Read the model definition and answer for the solid it produces. Units are mm, in the model's axes. Give positions to 0.01 mm unless a question says otherwise; leave off trailing zeros. Order: outer loops, then holes, each group sorted by start corner. A loop starts at its lowest first (then second) coordinate and runs counter-clockwise, first axis right, second up. Notation, with made-up numbers: M 76.25,-4 L 105.25,-4 A29 cw 105.25,35 Z; hole C 83,13.5 d5. An arc over 180 degrees is marked long. Write item = value, one per line. Start each with the question number.
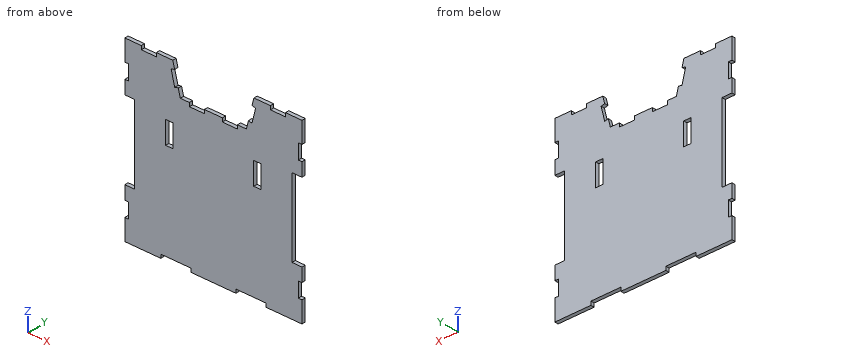
from build123d import *

# Parameters (mm, degrees)
CROQUIS1_W              = 4.84
CROQUIS1_H              = 15
SALIENTE_EXTRUIR1_DEPTH = 2.44


with BuildPart() as part:
    # Croquis1 → Saliente-Extruir1 (new body)
    with BuildSketch(Plane(origin=(0, 0, 0), x_dir=(1, 0, 0), z_dir=(0, 1, 0))):
        Polygon((-59, 45), (-59, 59), (-35, 59), (-35, 56.56), (-15, 56.56), (-15, 59), (15, 59), (15, 56.56), (35, 56.56), (35, 59), (59, 59), (59, 45), (56.56, 45), (56.56, 35), (59, 35), (59, 26), (52.4, 26), (52.4, -26), (59, -26), (59, -35), (56.56, -35), (56.56, -45), (59, -45), (59, -59), (48, -59), (48, -56.56), (38, -56.56), (38, -59), (27, -59), (25.787321875, -54.149287499), (28.154469575, -53.557500574), (25.729113325, -43.856075573), (23.361965624, -44.447862498), (22, -39), (16, -39), (16, -36.56), (6, -36.56), (6, -39), (-6, -39), (-6, -36.56), (-16, -36.56), (-16, -39), (-22, -39), (-23.361965624, -44.447862498), (-25.729113325, -43.856075573), (-28.154469575, -53.557500574), (-25.787321875, -54.149287499), (-27, -59), (-38, -59), (-38, -56.56), (-48, -56.56), (-48, -59), (-59, -59), (-59, -45), (-56.56, -45), (-56.56, -35), (-59, -35), (-59, -26), (-52.4, -26), (-52.4, 26), (-59, 26), (-59, 35), (-56.56, 35), (-56.56, 45), align=None)
        with Locations((29.32, -15.28)):
            Rectangle(CROQUIS1_W, CROQUIS1_H, mode=Mode.SUBTRACT)
        with Locations((-29.32, -15.28)):
            Rectangle(CROQUIS1_W, CROQUIS1_H, mode=Mode.SUBTRACT)
    extrude(amount=SALIENTE_EXTRUIR1_DEPTH)


solid = part.part
1) Find section C-C on x = -44.5. Determine the outline of the cut face in (y, z).
2) Find the intervals of material crossed by probe 1 along X at (y, z) = (2.15, 10); probe 2 along X at (y, z) = (0.1, 5); probe 3 along Z at (x, y) = (15.5, 1.75), in increasing order. Write a range as [from, to].
3) Find section D-D on y = 1.6. Count the separate pieces of the cut face and the enclosed holes in it, plus the area to 3 significant figures.
4) Find section A-A on x = -30. Determine the outline of the cut face in (y, z), plus the area to 3 significant figures.
5) Each of these flat-tipped pins is pushed along its axis until it touches: P1, Ø0.7, axis at x = -44.5, y = 1.5, coming from the +Z side; P2, Ø2, axis at x = 32, z = -42, coming from the -Y side; P3, Ø0.7, axis at y = 1.5, z = -41.5, coming from the -X side. Where does it stop, or does it pass through?
6) Find section B-B on z = -41. Determine the outline of the cut face in (x, y).
Numbers:
q1.outline = M 0,-59 L 2.44,-59 L 2.44,56.56 L 0,56.56 Z
q2.probe_1 = [-52.4, -31.74], [-26.9, 26.9], [31.74, 52.4]
q2.probe_2 = [-52.4, 52.4]
q2.probe_3 = [-56.56, 36.56]
q3.separate_pieces = 1
q3.enclosed_holes = 2
q3.area = 11,800 mm2
q4.outline = M 0,-56.56 L 2.44,-56.56 L 2.44,7.78 L 0,7.78 Z; M 0,22.78 L 2.44,22.78 L 2.44,59 L 0,59 Z
q4.area = 245 mm2
q5.P1 = 56.56
q5.P2 = 0
q5.P3 = -56.56
q6.outline = M -56.56,0 L 56.56,0 L 56.56,2.44 L -56.56,2.44 Z
